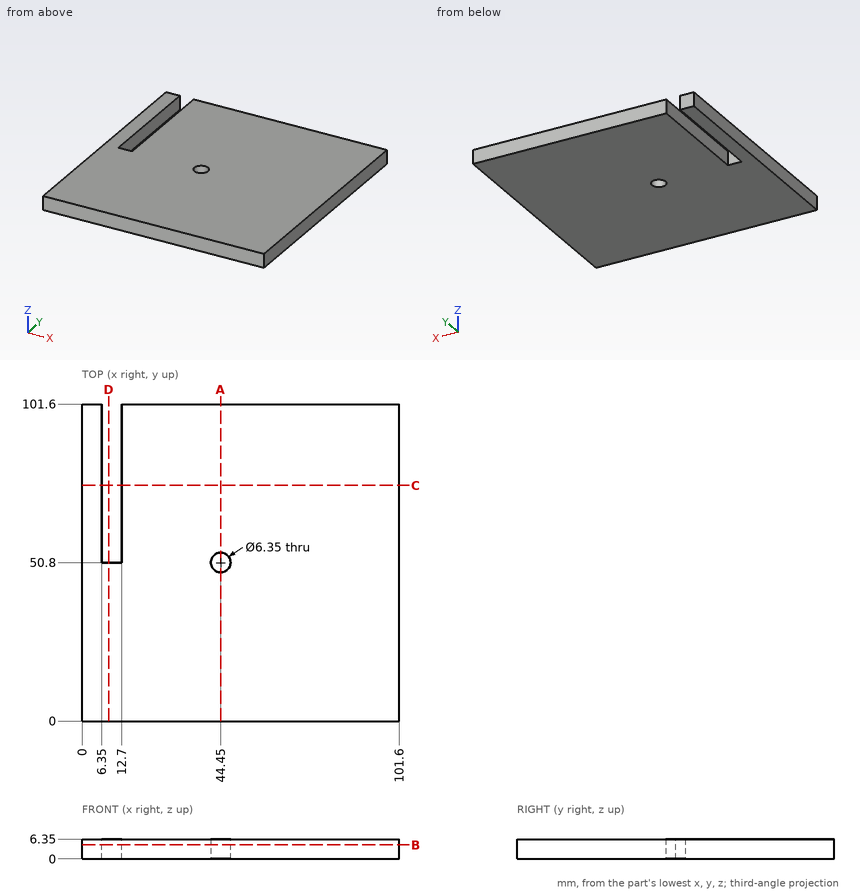
The drawing under review shows one solid part. Ordinate dimensions are in mm from its lowest x, y, z. Coordinates: 2 decimals unless noted, no trailing zeros. Order: outer loops, then holes, each group sorted by start corner. A loop starts at its lowest first (then second) coordinate and runs counter-clockwise, first axis right, second up. Notation, with made-up numbers: (22, 36.25) -> (37, 36.25) arc R18 cw to (37, 47.25) -> close; hole circle Ø11 at (33, -2.5). An arc over 180 degrees is marked (long way). Answer in a Markdown table with one row per item.
(1) Wall thickness on line 1 along X through (y, z) = (63, 1); line 2 along Y through (x, z) = (44.45, 1.5) (3 decimals); line 3 along Y through (x, z) = (11, 2): over which ranges is each line inside the solid? List them lowest first.
Answers:
| item | result |
|---|---|
| line 1 | 0 to 6.35, 12.7 to 101.6 |
| line 2 | 0 to 47.625, 53.975 to 101.6 |
| line 3 | 0 to 50.8 |
(2) Consider section B-B (z = 4.5). Write out the cut boundary in (x, y) (3 decimals), plus the area to 3 significant figures.
Answers:
| item | result |
|---|---|
| outline | (0, 0) -> (101.6, 0) -> (101.6, 101.6) -> (12.7, 101.6) -> (12.7, 50.8) -> (6.35, 50.8) -> (6.35, 101.6) -> (0, 101.6) -> close; hole circle Ø6.35 at (44.45, 50.8) |
| area | 9,970 mm² |
(3) Insertion check: pin 1 (1 mm diameter, centred on x = 89, z = 5.5, fed in from -Y). The pin has a flat end and moves straight along its axis. Give the tip position at first contact, or say it passes through.
Answers:
| item | result |
|---|---|
| pin 1 | y = 0 |
(4) Consider section C-C (y = 75.5). Write out the cut boundary in (x, z).
Answers:
| item | result |
|---|---|
| outline | (0, 0) -> (6.35, 0) -> (6.35, 6.35) -> (0, 6.35) -> close; (12.7, 0) -> (101.6, 0) -> (101.6, 6.35) -> (12.7, 6.35) -> close |
(5) Consider section A-A (x = 44.45). Write out the cut boundary in (y, z) (3 decimals), plus the area to 3 significant figures.
Answers:
| item | result |
|---|---|
| outline | (0, 0) -> (47.625, 0) -> (47.625, 6.35) -> (0, 6.35) -> close; (53.975, 0) -> (101.6, 0) -> (101.6, 6.35) -> (53.975, 6.35) -> close |
| area | 605 mm² |
(6) Consider section D-D (x = 8.5). Write out the cut boundary in (y, z).
Answers:
| item | result |
|---|---|
| outline | (0, 0) -> (50.8, 0) -> (50.8, 6.35) -> (0, 6.35) -> close |
